Source: CAD feature listing. Evaluate the final solid. Frame: model axes, mm. Face numbers are marked on the shaded views. Coordinates: 2 decimals unless noted, no trailing zeros. Order: outer loops, then holes, each group sorted by start corner. A loop starts at its lowest first (then second) coordinate and runs counter-clockwise, first axis right, second up.
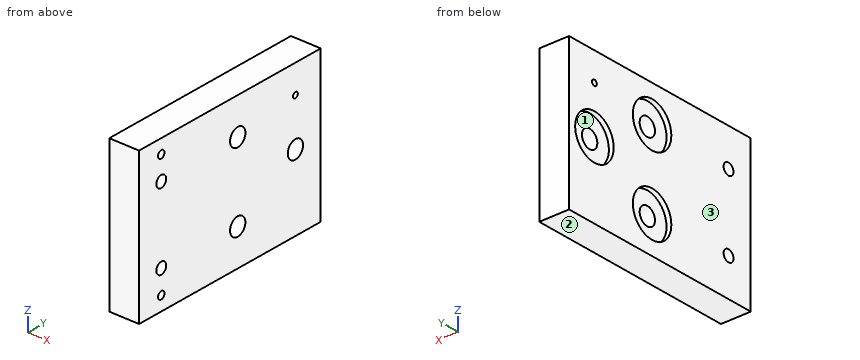
```python
from build123d import *

# Parameters (mm, degrees)
SKETCH26_W                                          = 6.35
SKETCH26_H                                          = 32
BOSS_EXTRUDE2_DEPTH                                 = 45
CUT_EXTRUDE7_REACH                                  = 8.35
SKETCH27_R                                          = 1.595
CBORE_FOR_6_BINDING_HEAD_MACHINE_SCREW1_D           = 3.7973
CBORE_FOR_6_BINDING_HEAD_MACHINE_SCREW1_DEPTH       = 46.5
CBORE_FOR_6_BINDING_HEAD_MACHINE_SCREW1_CBORE_D     = 9.525
CBORE_FOR_6_BINDING_HEAD_MACHINE_SCREW1_CBORE_DEPTH = 1.016
CBORE_FOR_6_BINDING_HEAD_MACHINE_SCREW1_TIP         = 1.140824014
F_0_80_TAPPED_HOLE1_D                               = 1.19126
F_2_CLEARANCE_HOLE1_D                               = 2.4384
F_2_CLEARANCE_HOLE1_DEPTH                           = 20.32
F_2_CLEARANCE_HOLE1_TIP                             = 0.732569267
F_1_16_0_0625_DOWEL_HOLE1_D                         = 1.5875
F_1_16_0_0625_DOWEL_HOLE1_DEPTH                     = 3.523066884
F_1_16_0_0625_DOWEL_HOLE1_TIP                       = 0.476933116


with BuildPart() as part:
    # Sketch26 → Boss-Extrude2 (new body)
    with BuildSketch(Plane(origin=(0, 0, 0), x_dir=(-1, 0, 0), z_dir=(0, 1, 0))):
        with Locations((-3.175, 16)):
            Rectangle(SKETCH26_W, SKETCH26_H)
    extrude(amount=BOSS_EXTRUDE2_DEPTH)

    # Sketch27 → Cut-Extrude7 (cut, up to next)
    with BuildSketch(Plane.ZY, mode=Mode.PRIVATE) as cut_extrude7_sk1:
        with Locations((16, 38.725)):
            Circle(SKETCH27_R)
    cut_extrude7_tool1 = extrude(cut_extrude7_sk1.sketch, amount=-CUT_EXTRUDE7_REACH, mode=Mode.PRIVATE) & part.part
    add(cut_extrude7_tool1.solids().sort_by_distance((0, 38.725, 16))[0], mode=Mode.SUBTRACT)
    # Sketch27 → Cut-Extrude7 (cut, up to next)
    with BuildSketch(Plane.ZY, mode=Mode.PRIVATE) as cut_extrude7_sk2:
        with Locations((24.248891971, 24.4375)):
            Circle(SKETCH27_R)
    cut_extrude7_tool2 = extrude(cut_extrude7_sk2.sketch, amount=-CUT_EXTRUDE7_REACH, mode=Mode.PRIVATE) & part.part
    add(cut_extrude7_tool2.solids().sort_by_distance((0, 24.4375, 24.248892))[0], mode=Mode.SUBTRACT)
    # Sketch27 → Cut-Extrude7 (cut, up to next)
    with BuildSketch(Plane.ZY, mode=Mode.PRIVATE) as cut_extrude7_sk3:
        with Locations((7.751108029, 24.4375)):
            Circle(SKETCH27_R)
    cut_extrude7_tool3 = extrude(cut_extrude7_sk3.sketch, amount=-CUT_EXTRUDE7_REACH, mode=Mode.PRIVATE) & part.part
    add(cut_extrude7_tool3.solids().sort_by_distance((0, 24.4375, 7.751108))[0], mode=Mode.SUBTRACT)

    # CBORE for #6 Binding Head Machine Screw1
    with Locations(Plane.ZY):
        with Locations((16, 38.725), (24.248891971, 24.4375), (7.751108029, 24.4375)):
            CounterBoreHole(CBORE_FOR_6_BINDING_HEAD_MACHINE_SCREW1_D / 2, CBORE_FOR_6_BINDING_HEAD_MACHINE_SCREW1_CBORE_D / 2, CBORE_FOR_6_BINDING_HEAD_MACHINE_SCREW1_CBORE_DEPTH, depth=CBORE_FOR_6_BINDING_HEAD_MACHINE_SCREW1_DEPTH)
            with Locations((0, 0, -(CBORE_FOR_6_BINDING_HEAD_MACHINE_SCREW1_DEPTH + CBORE_FOR_6_BINDING_HEAD_MACHINE_SCREW1_TIP / 2))):  # 118° drill point
                Cone(0, CBORE_FOR_6_BINDING_HEAD_MACHINE_SCREW1_D / 2, CBORE_FOR_6_BINDING_HEAD_MACHINE_SCREW1_TIP, mode=Mode.SUBTRACT)

    # #0-80 Tapped Hole1 (through all)
    with Locations(Plane.ZY):
        with Locations((26, 38.725)):
            Hole(F_0_80_TAPPED_HOLE1_D / 2)

    # #2 Clearance Hole1
    with Locations(Plane.ZY):
        with Locations((8, 5.5), (24, 5.5)):
            Hole(F_2_CLEARANCE_HOLE1_D / 2, depth=F_2_CLEARANCE_HOLE1_DEPTH)
            with Locations((0, 0, -(F_2_CLEARANCE_HOLE1_DEPTH + F_2_CLEARANCE_HOLE1_TIP / 2))):  # 118° drill point
                Cone(0, F_2_CLEARANCE_HOLE1_D / 2, F_2_CLEARANCE_HOLE1_TIP, mode=Mode.SUBTRACT)

    # 1/16 (0.0625) Dowel Hole1
    with Locations(Plane(origin=(6.35, 0, 0), x_dir=(0, 0, -1), z_dir=(1, 0, 0))):
        with Locations((-29, 5.5), (-3, 5.5)):
            Hole(F_1_16_0_0625_DOWEL_HOLE1_D / 2, depth=F_1_16_0_0625_DOWEL_HOLE1_DEPTH)
            with Locations((0, 0, -(F_1_16_0_0625_DOWEL_HOLE1_DEPTH + F_1_16_0_0625_DOWEL_HOLE1_TIP / 2))):  # 118° drill point
                Cone(0, F_1_16_0_0625_DOWEL_HOLE1_D / 2, F_1_16_0_0625_DOWEL_HOLE1_TIP, mode=Mode.SUBTRACT)


solid = part.part
```
Q1. Section query B-B on z = 8. Output: boundary loops of the cut face in (x, y), plus the area to 3 significant figures.
Solutions:
outline: (0, 0) - (6.35, 0) - (6.35, 4.28) - (0, 4.28) - close; (0, 6.72) - (6.35, 6.72) - (6.35, 22.56) - (1.02, 22.56) - (1.02, 19.68) - (0, 19.68) - close; (0, 29.19) - (1.02, 29.19) - (1.02, 26.32) - (6.35, 26.32) - (6.35, 45) - (0, 45) - close
area: 241 mm2
Q2. Section query C-C on x = 4.5. Give the number of separate pieces and of enclosed holes in the cut face, plus the area to 3 significant figures.
Solutions:
separate pieces: 1
enclosed holes: 8
area: 1,390 mm2
Q3. Pin query (flat end, axial travel): P1, Ø2, axis at y = 23, z = 9.5, coming from the -X side. Return the tip coordinate at first contact, or that it passes through.
Solutions:
P1: stops at x = 1.02
Q4. Material intervals for line 1 along Y through (x, z) = (6, 3); line 2 along Z through (x, y) = (2.5, 6); line 3 along Z through (x, y) = (3.25, 38.5), sorted ascending.
Solutions:
line 1: y = 0 to 4.71, 6.29 to 45
line 2: z = 0 to 6.89, 9.11 to 22.89, 25.11 to 32
line 3: z = 0 to 14.11, 17.89 to 25.45, 26.55 to 32
Q5. Section query A-A on z = 16. Output: boundary loops of the cut face in (x, y), plus the area to 3 significant figures.
Solutions:
outline: (0, 0) - (6.35, 0) - (6.35, 36.83) - (1.02, 36.83) - (1.02, 33.96) - (0, 33.96) - close; (0, 43.49) - (1.02, 43.49) - (1.02, 40.62) - (6.35, 40.62) - (6.35, 45) - (0, 45) - close
area: 256 mm2
Q6. Section query D-D on y = 28. Output: boundary loops of the cut face in (x, z), plus the area to 3 significant figures.
Solutions:
outline: (0, 0) - (6.35, 0) - (6.35, 32) - (0, 32) - (0, 27.41) - (1.02, 27.41) - (1.02, 21.09) - (0, 21.09) - (0, 10.91) - (1.02, 10.91) - (1.02, 4.59) - (0, 4.59) - close
area: 190 mm2
Q7. Pull-direction query (Z, two-part tool) for the marked faces 1, 2 and 3; classes: pulls with the +Z half, pulls with the -Z half, needs draft (parallel to the pull), parting line crosses it, or undercut.
Solutions:
face 1: undercut
face 2: pulls with the -Z half
face 3: needs draft
